Read the model definition and answer for the solid it produces. Units are mm, in the model's axes. A direction names the side the tool comes from. Give positions to 0.01 mm unless a question says otherwise; leave off trailing zeros. Order: outer loops, then holes, each group sorted by start corner. A loop starts at its lowest first (then second) coordinate and runs counter-clockwise, first axis right, second up. Notation, with made-up numbers: (57.5, 61.25) - (78.5, 61.25) arc R30 ccw to (78.5, 90.25) - close; hole circle Ø2 at (-15.75, 75.5). An arc over 180 degrees is marked (long way). Use a Markdown table: item, result. Add a question column.
1. Consider L1, parallel to X at y = 5.5, z = -17.5; L2, parallel to Z at x = 31, y = 31. Determine where each line is inside the solid, lowest interval first.
2. Which of the six approach directions +Z, -Z, +X, -X, +Y, -Y give full straight-line access (tool end or side, diameter ignored) to faces 1 (the flat face through (25, 30, -1)), 2 (the flat face through (21, 30, -55)), 3 (the flat face through (14, 30, -53))?
3. A cutting plane is placed at A-A on x = 21. Determine the outline of the cut face in (y, z), and give its area (3 significant figures).
4. A cutting plane is placed at D-D on z = -24.5. Determine the outline of the cut face in (x, y).
5. For a pull along Z with two mould halves and no side action, classify faces 4 (the flat face through (14, 30, -2)), 5 (the flat face through (14, 30, 0)), 6 (the flat face through (35, 30, -28)) as released by +Z, released by -Z, zero draft, split by the parting line, or undercut.
6. A cutting plane is placed at B-B on x = 26.5. Determine the outline of the cut face in (y, z), and give its area (3 significant figures).
7. A cutting plane is placed at C-C on y = 48.5. Determine the outline of the cut face in (x, z), and give its area (3 significant figures).
```python
from build123d import *

# Parameters (mm, degrees)
SKETCH1_W           = 31
SKETCH1_H           = 51
BOSS_EXTRUDE1_DEPTH = 60
CUT_EXTRUDE1_DEPTH  = 60


with BuildPart() as part:
    # Sketch1 → Boss-Extrude1 (new body)
    with BuildSketch(Plane(origin=(0, 0, 0), x_dir=(1, 0, 0), z_dir=(0, 1, 0))):
        with BuildLine():
            Line((0, 1), (0, 54))
            ThreePointArc((0, 54), (0.292893219, 54.707106781), (1, 55))
            Line((1, 55), (34, 55))
            ThreePointArc((34, 55), (34.707106781, 54.707106781), (35, 54))
            Line((35, 54), (35, 1))
            ThreePointArc((35, 1), (34.707106781, 0.292893219), (34, 0))
            Line((34, 0), (1, 0))
            ThreePointArc((1, 0), (0.292893219, 0.292893219), (0, 1))
        make_face()
        with Locations((17.5, 27.5)):
            Rectangle(SKETCH1_W, SKETCH1_H, mode=Mode.SUBTRACT)
    extrude(amount=BOSS_EXTRUDE1_DEPTH)

    # Sketch3 → Cut-Extrude1 (cut)
    with BuildSketch(Plane.XY):
        with BuildLine():
            Line((15.5, 54), (15.5, 6))
            ThreePointArc((15.5, 6), (17.5, 4), (19.5, 6))
            Line((19.5, 6), (19.5, 54))
            ThreePointArc((19.5, 54), (17.5, 56), (15.5, 54))
        make_face()
        with BuildLine():
            Line((28, 44), (28, 16))
            ThreePointArc((28, 16), (26.5, 14.5), (25, 16))
            Line((25, 16), (25, 44))
            ThreePointArc((25, 44), (26.5, 45.5), (28, 44))
        make_face()
        with BuildLine():
            Line((7, 44), (7, 16))
            ThreePointArc((7, 16), (8.5, 14.5), (10, 16))
            Line((10, 16), (10, 44))
            ThreePointArc((10, 44), (8.5, 45.5), (7, 44))
        make_face()
    extrude(amount=-CUT_EXTRUDE1_DEPTH, mode=Mode.SUBTRACT)


solid = part.part
```
Output values:
| question | item | result |
|---|---|---|
| 1 | L1 | 0 to 2, 33 to 35 |
| 1 | L2 | -55 to -53, -2 to 0 |
| 2 | face 1 | +Z, -Z |
| 2 | face 2 | -Z, +X, -X, +Y, -Y |
| 2 | face 3 | +Y, -Y |
| 3 | outline | (0, -55) - (60, -55) - (60, -53) - (0, -53) - close; (0, -2) - (60, -2) - (60, 0) - (0, 0) - close |
| 3 | area | 240 mm² |
| 4 | outline | (0, 0) - (2, 0) - (2, 60) - (0, 60) - close; (33, 0) - (35, 0) - (35, 60) - (33, 60) - close |
| 5 | face 4 | undercut |
| 5 | face 5 | released by +Z |
| 5 | face 6 | zero draft |
| 6 | outline | (0, -55) - (14.5, -55) - (14.5, -53) - (0, -53) - close; (0, -2) - (14.5, -2) - (14.5, 0) - (0, 0) - close; (45.5, -55) - (60, -55) - (60, -53) - (45.5, -53) - close; (45.5, -2) - (60, -2) - (60, 0) - (45.5, 0) - close |
| 6 | area | 116 mm² |
| 7 | outline | (0, -54) arc R1 ccw to (1, -55) - (15.5, -55) - (15.5, -53) - (2, -53) - (2, -2) - (15.5, -2) - (15.5, 0) - (1, 0) arc R1 ccw to (0, -1) - close; (19.5, -55) - (34, -55) arc R1 ccw to (35, -54) - (35, -1) arc R1 ccw to (34, 0) - (19.5, 0) - (19.5, -2) - (33, -2) - (33, -53) - (19.5, -53) - close |
| 7 | area | 327 mm² |
